from build123d import *

# Parameters (mm, degrees)
F0_R     = 1.6
F1_DEPTH = 3


with BuildPart() as f1:
    # F0 (on Top) → F1 (new body)
    with BuildSketch(Plane.XY):
        with BuildLine():
            ThreePointArc((-0.5, 23), (0, 22.5), (0.5, 23))
            Line((0.5, 23), (-0.5, 23))
        make_face()
        with BuildLine():
            Line((-0.5, 23), (0.5, 23))
            ThreePointArc((0.5, 23), (0, 23.5), (-0.5, 23))
        make_face()
        with BuildLine():
            Line((30.5, 23), (0.5, 23))
            ThreePointArc((0.5, 23), (0, 22.5), (-0.5, 23))
            Line((-0.5, 23), (-30.5, 23))
            Line((-30.5, 23), (-30.5, -23))
            Line((-30.5, -23), (30.5, -23))
            Line((30.5, -23), (30.5, 23))
        make_face()
        with Locations((-26.3, -13.8)):
            Circle(F0_R, mode=Mode.SUBTRACT)
        with Locations((26.3, -13.8)):
            Circle(F0_R, mode=Mode.SUBTRACT)
        with Locations((-26.3, 13.8)):
            Circle(F0_R, mode=Mode.SUBTRACT)
        with Locations((26.3, 13.8)):
            Circle(F0_R, mode=Mode.SUBTRACT)
    extrude(amount=F1_DEPTH)


solid = f1.part
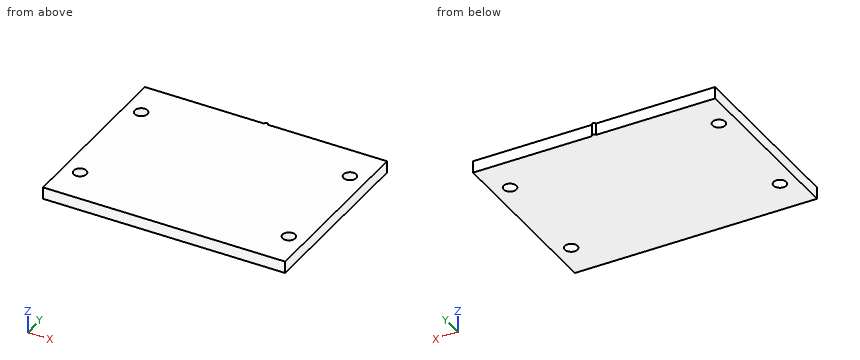
Can you work these out from the model? Positions are in its coordinate system, mm. Give positions to 0.01 mm unless a question says otherwise; leave off trailing zeros. Loops run counter-clockwise (first coordinate to the right, second up) from the corner with the lowest first, then second, coordinate; pieces in that order, holes last. Notation, with made-up numbers: (-9.75, -20.75) -> (-3.75, -20.75) arc R19 ccw to (-3.75, -12.75) -> close; hole circle Ø6 at (25, -12.75). An arc over 180 degrees is marked (long way). Return JSON: item names as keys, results as strings.
Q1. I want a section at B-B, the plane z = 0.7. List the corners of the cut face in (x, y) for me.
Checks:
{"outline": "(-30.5, -23) -> (30.5, -23) -> (30.5, 23) -> (0.5, 23) arc R0.5 ccw to (-0.5, 23) -> (-30.5, 23) -> close; hole circle Ø3.2 at (-26.3, -13.8); hole circle Ø3.2 at (-26.3, 13.8); hole circle Ø3.2 at (26.3, -13.8); hole circle Ø3.2 at (26.3, 13.8)"}
Q2. I want a section at C-C, the plane x = 26.3. List the corners of the cut face in (y, z) for me.
Checks:
{"outline": "(-23, 0) -> (-15.4, 0) -> (-15.4, 3) -> (-23, 3) -> close; (-12.2, 0) -> (12.2, 0) -> (12.2, 3) -> (-12.2, 3) -> close; (15.4, 0) -> (23, 0) -> (23, 3) -> (15.4, 3) -> close"}
Q3. I need wall thicknesses on probe 1 along Y at (x, z) = (26.3, 1.05); probe 2 along Y at (x, z) = (-25, 2.7); probe 3 along Y at (x, z) = (23, 0.75). Which ranges of each line are inside material? Lowest first, please.
Checks:
{"probe 1": "y = -23 to -15.4, -12.2 to 12.2, 15.4 to 23", "probe 2": "y = -23 to -14.73, -12.87 to 12.87, 14.73 to 23", "probe 3": "y = -23 to 23"}
Q4. For pin 1 Ø1 at (x, z) = (2, 2.5) entering from +Y, with a flat end and sliding along its axis, tell me the tip position at first contact or that it passes through.
Checks:
{"pin 1": "stops at y = 23"}
Q5. I want a section at A-A, the plane y = 13.8. List the corners of the cut face in (x, z) for me, then the cut area to 3 significant figures.
Checks:
{"outline": "(-30.5, 0) -> (-27.9, 0) -> (-27.9, 3) -> (-30.5, 3) -> close; (-24.7, 0) -> (24.7, 0) -> (24.7, 3) -> (-24.7, 3) -> close; (27.9, 0) -> (30.5, 0) -> (30.5, 3) -> (27.9, 3) -> close", "area": "164 mm2"}
